The model under review builds one solid part; all positions refer to its coordinate system, in mm. Face numbers are marked on the shaded views. A direction names the side the tool comes from. Coordinates: 2 decimals unless noted, no trailing zeros. Write each loop counter-clockwise with the first axis right and the second up, starting at its lowest first coordinate (ties: lowest second). Pieces come first, ordered by that corner, then holes.
1) Machinability: for the marked faces 3, 4, 5, 6 and 7, which of the approach directions +Z, -Z, +X, -X, +Y, -Y give a long, thin tool a straight path to every point of the face, cutting with its end or side? Answer none if there is none.
2) For P1, Ø3, axis at x = 90, y = -19, coming from the -Z side; P2, Ø0.9, axis at y = 5.5, z = 3, coming from the -X side; P3, Ø14.5, axis at x = 138, y = -5, coming from the -Z side; P4, Ø5.5, axis at x = 166.5, y = -2, coming from the +Z side, all flat-tipped, find the tip position at first contact; note any pin that passes through.
3) Add section B-B, the plane x = 50. State the section outline as (y, z) points, then the cut area to 3 significant figures.
4) Add section A-A, the plane x = 18. State the section outline as (y, z) points, then the cut area to 3 significant figures.
5) Mouldability with a two-part tool opening along X and no side actions: class the marked faces 1 and 2 as released by +X, released by -X, zero draft, split by the parting line, or undercut.
6) Add section C-C, the plane y = 0. Give the number of separate pieces and of enclosed holes in the cut face, then the cut area to 3 significant figures.
7) For line 1 (X direction, y = -19, z = 3.8); line 2 (X direction, y = 1, z = 0.95); line 3 (Y direction, x = -20, z = 0.4), list the stretches that pass through material, from the lowest coordinate up.
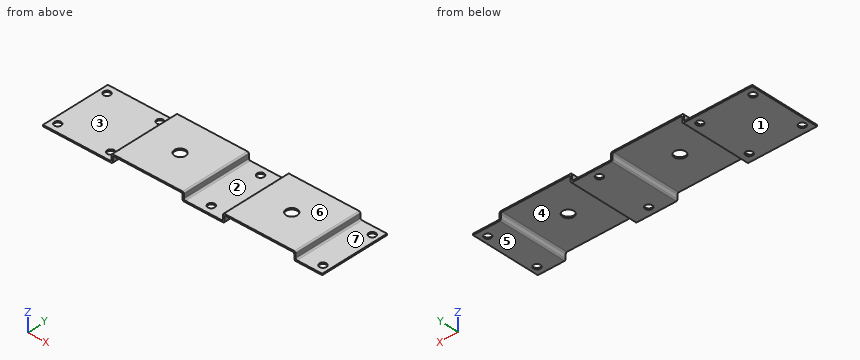
from build123d import *

# Parameters (mm, degrees)
SKETCH1_W           = 50
SKETCH1_H           = 50
BOSS_EXTRUDE1_DEPTH = 1
BOSS_EXTRUDE2_START = 5
SKETCH2_W           = 50
SKETCH2_H           = 50
BOSS_EXTRUDE2_DEPTH = 1
SKETCH3_W           = 30
SKETCH3_H           = 50
BOSS_EXTRUDE3_DEPTH = 1
BOSS_EXTRUDE4_START = 5
SKETCH4_W           = 50
SKETCH4_H           = 50
BOSS_EXTRUDE4_DEPTH = 1
SKETCH5_W           = 20
SKETCH5_H           = 50
BOSS_EXTRUDE5_DEPTH = 1
SKETCH6_W           = 6
SKETCH6_H           = 50
BOSS_EXTRUDE6_DEPTH = 1
SKETCH7_W           = 6
SKETCH7_H           = 50
BOSS_EXTRUDE7_DEPTH = 1
SKETCH8_W           = 6
SKETCH8_H           = 50
BOSS_EXTRUDE8_DEPTH = 1
SKETCH9_W           = 6
SKETCH9_H           = 50
BOSS_EXTRUDE9_DEPTH = 1
FILLET1_R           = 1
FILLET2_R           = 1
FILLET3_R           = 1
FILLET4_R           = 1
FILLET5_R           = 1
FILLET6_R           = 1
FILLET7_R           = 1
FILLET8_R           = 1
FILLET9_R           = 1
FILLET10_R          = 1
FILLET11_R          = 1
FILLET12_R          = 1
FILLET13_R          = 1
FILLET14_R          = 1
FILLET15_R          = 1
FILLET16_R          = 1
SKETCH10_R          = 2.5
CUT_EXTRUDE1_DEPTH  = 1
SKETCH11_R          = 4
SKETCH11_R_2        = 2.5
CUT_EXTRUDE7_DEPTH  = 50.5


with BuildPart() as part:
    # Sketch1 → Boss-Extrude1 (new body)
    with BuildSketch(Plane.XY):
        Rectangle(SKETCH1_W, SKETCH1_H)
    extrude(amount=BOSS_EXTRUDE1_DEPTH)



with BuildPart() as body_2:
    # Sketch2 → Boss-Extrude2 (new body)
    with BuildSketch(Plane.XY.offset(BOSS_EXTRUDE2_START)):
        with Locations((50, 0)):
            Rectangle(SKETCH2_W, SKETCH2_H)
    extrude(amount=BOSS_EXTRUDE2_DEPTH)


with BuildPart() as body_3:
    # Sketch3 → Boss-Extrude3 (new body)
    with BuildSketch(Plane.XY):
        with Locations((90, 0)):
            Rectangle(SKETCH3_W, SKETCH3_H)
    extrude(amount=BOSS_EXTRUDE3_DEPTH)


with BuildPart() as body_4:
    # Sketch4 → Boss-Extrude4 (new body)
    with BuildSketch(Plane.XY.offset(BOSS_EXTRUDE4_START)):
        with Locations((130, 0)):
            Rectangle(SKETCH4_W, SKETCH4_H)
    extrude(amount=BOSS_EXTRUDE4_DEPTH)


with BuildPart() as body_5:
    # Sketch5 → Boss-Extrude5 (new body)
    with BuildSketch(Plane.XY):
        with Locations((165, 0)):
            Rectangle(SKETCH5_W, SKETCH5_H)
    extrude(amount=BOSS_EXTRUDE5_DEPTH)


with BuildPart() as part_1:
    add(part.part)

    add(body_2.part)  # Boss-Extrude6 merges body 2
    # Sketch6 → Boss-Extrude6 (add)
    with BuildSketch(Plane.ZY.offset(-25)):
        with Locations((3, 0)):
            Rectangle(SKETCH6_W, SKETCH6_H)
    extrude(amount=BOSS_EXTRUDE6_DEPTH)


    add(body_3.part)  # Boss-Extrude7 merges body 3
    # Sketch7 → Boss-Extrude7 (add)
    with BuildSketch(Plane(origin=(75, 0, 0), x_dir=(0, 0, -1), z_dir=(1, 0, 0))):
        with Locations((-3, 0)):
            Rectangle(SKETCH7_W, SKETCH7_H)
    extrude(amount=BOSS_EXTRUDE7_DEPTH)


    add(body_4.part)  # Boss-Extrude8 merges body 4
    # Sketch8 → Boss-Extrude8 (add)
    with BuildSketch(Plane.ZY.offset(-105)):
        with Locations((3, 0)):
            Rectangle(SKETCH8_W, SKETCH8_H)
    extrude(amount=BOSS_EXTRUDE8_DEPTH)


    add(body_5.part)  # Boss-Extrude9 merges body 5
    # Sketch9 → Boss-Extrude9 (add)
    with BuildSketch(Plane(origin=(155, 0, 0), x_dir=(0, 0, -1), z_dir=(1, 0, 0))):
        with Locations((-3, 0)):
            Rectangle(SKETCH9_W, SKETCH9_H)
    extrude(amount=BOSS_EXTRUDE9_DEPTH)

    # Fillet1
    fillet1_edges = [part_1.edges().sort_by_distance(p)[0] for p in [
        (24, 0, 1),
    ]]
    fillet(fillet1_edges, radius=FILLET1_R)

    # Fillet2
    fillet2_edges = [part_1.edges().sort_by_distance(p)[0] for p in [
        (24, 0, 6),
    ]]
    fillet(fillet2_edges, radius=FILLET2_R)

    # Fillet3
    fillet3_edges = [part_1.edges().sort_by_distance(p)[0] for p in [
        (76, 0, 6),
    ]]
    fillet(fillet3_edges, radius=FILLET3_R)

    # Fillet4
    fillet4_edges = [part_1.edges().sort_by_distance(p)[0] for p in [
        (76, 0, 1),
    ]]
    fillet(fillet4_edges, radius=FILLET4_R)

    # Fillet5
    fillet5_edges = [part_1.edges().sort_by_distance(p)[0] for p in [
        (104, 0, 6),
    ]]
    fillet(fillet5_edges, radius=FILLET5_R)

    # Fillet6
    fillet6_edges = [part_1.edges().sort_by_distance(p)[0] for p in [
        (104, 0, 1),
    ]]
    fillet(fillet6_edges, radius=FILLET6_R)

    # Fillet7
    fillet7_edges = [part_1.edges().sort_by_distance(p)[0] for p in [
        (156, 0, 6),
    ]]
    fillet(fillet7_edges, radius=FILLET7_R)

    # Fillet8
    fillet8_edges = [part_1.edges().sort_by_distance(p)[0] for p in [
        (156, 0, 1),
    ]]
    fillet(fillet8_edges, radius=FILLET8_R)

    # Fillet9
    fillet9_edges = [part_1.edges().sort_by_distance(p)[0] for p in [
        (155, 0, 0),
    ]]
    fillet(fillet9_edges, radius=FILLET9_R)

    # Fillet10
    fillet10_edges = [part_1.edges().sort_by_distance(p)[0] for p in [
        (155, 0, 5),
    ]]
    fillet(fillet10_edges, radius=FILLET10_R)

    # Fillet11
    fillet11_edges = [part_1.edges().sort_by_distance(p)[0] for p in [
        (105, 0, 5),
    ]]
    fillet(fillet11_edges, radius=FILLET11_R)

    # Fillet12
    fillet12_edges = [part_1.edges().sort_by_distance(p)[0] for p in [
        (105, 0, 0),
    ]]
    fillet(fillet12_edges, radius=FILLET12_R)

    # Fillet13
    fillet13_edges = [part_1.edges().sort_by_distance(p)[0] for p in [
        (25, 0, 5),
    ]]
    fillet(fillet13_edges, radius=FILLET13_R)

    # Fillet14
    fillet14_edges = [part_1.edges().sort_by_distance(p)[0] for p in [
        (25, 0, 0),
    ]]
    fillet(fillet14_edges, radius=FILLET14_R)

    # Fillet15
    fillet15_edges = [part_1.edges().sort_by_distance(p)[0] for p in [
        (75, 0, 5),
    ]]
    fillet(fillet15_edges, radius=FILLET15_R)

    # Fillet16
    fillet16_edges = [part_1.edges().sort_by_distance(p)[0] for p in [
        (75, 0, 0),
    ]]
    fillet(fillet16_edges, radius=FILLET16_R)

    # Sketch10 → Cut-Extrude1 (cut)
    with BuildSketch(Plane.XY.offset(1)):
        with Locations((-20, 19)):
            Circle(SKETCH10_R)
        with Locations((-20, -19)):
            Circle(SKETCH10_R)
        with Locations((18, -19)):
            Circle(SKETCH10_R)
        with Locations((18, 19)):
            Circle(SKETCH10_R)
    extrude(amount=-CUT_EXTRUDE1_DEPTH, mode=Mode.SUBTRACT)

    # Sketch11 → Cut-Extrude7 (cut, symmetric)
    with BuildSketch(Plane.XY):
        with Locations(Location((50, 0, 0), (0, 0, 180))):
            Circle(SKETCH11_R)
        with Locations(Location((130, 0, 0), (0, 0, 180))):
            Circle(SKETCH11_R)
        with Locations(Location((90, 19, 0), (0, 0, 180))):
            Circle(SKETCH11_R_2)
        with Locations(Location((90, -19, 0), (0, 0, 180))):
            Circle(SKETCH11_R_2)
        with Locations(Location((170, 19, 0), (0, 0, 180))):
            Circle(SKETCH11_R_2)
        with Locations(Location((170, -19, 0), (0, 0, 180))):
            Circle(SKETCH11_R_2)
    extrude(amount=CUT_EXTRUDE7_DEPTH, both=True, mode=Mode.SUBTRACT)


solid = part_1.part
Geometry results:
1. face 3: +Z, -X, +Y, -Y
1. face 4: -Z, +Y, -Y
1. face 5: -Z, +X, -X, +Y, -Y
1. face 6: +Z, +X, -X, +Y, -Y
1. face 7: +Z, +X, +Y, -Y
2. P1: passes through
2. P2: stops at x = 24
2. P3: stops at z = 5
2. P4: stops at z = 1
3. outline: (-25, 5) - (-4, 5) - (-4, 6) - (-25, 6) - close; (4, 5) - (25, 5) - (25, 6) - (4, 6) - close
3. area: 42.0 mm2
4. outline: (-25, 0) - (-21.5, 0) - (-21.5, 1) - (-25, 1) - close; (-16.5, 0) - (16.5, 0) - (16.5, 1) - (-16.5, 1) - close; (21.5, 0) - (25, 0) - (25, 1) - (21.5, 1) - close
4. area: 40.0 mm2
5. face 1: zero draft
5. face 2: undercut
6. separate pieces: 3
6. enclosed holes: 0
6. area: 204 mm2
7. line 1: x = 24 to 25, 75 to 76, 104 to 105, 155 to 156
7. line 2: x = -25 to 25, 75 to 105, 155 to 175
7. line 3: y = -25 to -21.5, -16.5 to 16.5, 21.5 to 25
